```python
from build123d import *

# Parameters (mm, degrees)
BOX011_W          = 9.2
BOX011_H          = 10
BOX011_DEPTH      = 3.4
FILLET005_R       = 1
BOX010_W          = 5.2
BOX010_H          = 50
BOX010_DEPTH      = 1.6
BOX008_W          = 57.2
BOX008_H          = 38.2
BOX008_DEPTH      = 1.6
CYLINDER012_R     = 16.7
CYLINDER012_DEPTH = 1.6
CYLINDER011_R     = 19.9
CYLINDER011_DEPTH = 17
BOX007_W          = 77.1
BOX007_H          = 39.8
BOX007_DEPTH      = 17
CYLINDER010_R     = 21.5
CYLINDER010_DEPTH = 17
BOX006_W          = 78.7
BOX006_H          = 43
BOX006_DEPTH      = 17
FILLET002_R       = 2.4
CHAMFER005_SIZE   = 0.8
CHAMFER013_SIZE   = 0.8


with BuildPart() as usb:
    # Box011 → Box011 (new body)
    with BuildSketch(Plane(origin=(56.4, 45, 9.4), x_dir=(1, 0, 0), z_dir=(0, 0, 1))):
        with Locations((4.6, 5)):
            Rectangle(BOX011_W, BOX011_H)
    extrude(amount=BOX011_DEPTH)

    # Fillet005
    fillet005_edges = [usb.edges().sort_by_distance(p)[0] for p in [
        (56.4, 50, 12.8),
        (56.4, 50, 9.4),
        (65.6, 50, 12.8),
        (65.6, 50, 9.4),
    ]]
    fillet(fillet005_edges, radius=FILLET005_R)


with BuildPart() as obj1:
    # Box010 → Box010 (new body)
    with BuildSketch(Plane(origin=(37.9, 45, 13.8), x_dir=(1, 0, 0), z_dir=(0, 0, 1))):
        with Locations((2.6, 25)):
            Rectangle(BOX010_W, BOX010_H)
    extrude(amount=BOX010_DEPTH)


with BuildPart() as obj2:
    # Box008 → Box008 (new body)
    with BuildSketch(Plane(origin=(0, 50, 0), x_dir=(1, 0, 0), z_dir=(0, 0, 1))):
        with Locations((28.6, 19.1)):
            Rectangle(BOX008_W, BOX008_H)
    extrude(amount=BOX008_DEPTH)


with BuildPart() as zylinder012:
    # Cylinder012 → Cylinder012 (new body)
    with BuildSketch(Plane(origin=(76.2, 69.1, 0), x_dir=(1, 0, 0), z_dir=(0, 0, 1))):
        Circle(CYLINDER012_R)
    extrude(amount=CYLINDER012_DEPTH)


with BuildPart() as zylinder011:
    # Cylinder011 → Cylinder011 (new body)
    with BuildSketch(Plane(origin=(76.2, 69.1, 1.6), x_dir=(1, 0, 0), z_dir=(0, 0, 1))):
        Circle(CYLINDER011_R)
    extrude(amount=CYLINDER011_DEPTH)


with BuildPart() as fusion009:
    # Box007 → Box007 (new body)
    with BuildSketch(Plane(origin=(-0.8, 49.2, 1.6), x_dir=(1, 0, 0), z_dir=(0, 0, 1))):
        with Locations((38.55, 19.9)):
            Rectangle(BOX007_W, BOX007_H)
    extrude(amount=BOX007_DEPTH)

    # Fusion009: union Zylinder011
    add(zylinder011.part)


with BuildPart() as zylinder010:
    # Cylinder010 → Cylinder010 (new body)
    with BuildSketch(Plane(origin=(76.2, 69.1, 0), x_dir=(1, 0, 0), z_dir=(0, 0, 1))):
        Circle(CYLINDER010_R)
    extrude(amount=CYLINDER010_DEPTH)


with BuildPart() as top:
    # Box006 → Box006 (new body)
    with BuildSketch(Plane(origin=(-2.4, 47.6, 0), x_dir=(1, 0, 0), z_dir=(0, 0, 1))):
        with Locations((39.35, 21.5)):
            Rectangle(BOX006_W, BOX006_H)
    extrude(amount=BOX006_DEPTH)

    # Fusion008: union Zylinder010
    add(zylinder010.part)

    # Cut004: cut Fusion009
    add(fusion009.part, mode=Mode.SUBTRACT)

    # Fillet002
    fillet002_edges = [top.edges().sort_by_distance(p)[0] for p in [
        (-2.4, 47.6, 8.5),
        (-2.4, 90.6, 8.5),
    ]]
    fillet(fillet002_edges, radius=FILLET002_R)

    # Cut005: cut Zylinder012
    add(zylinder012.part, mode=Mode.SUBTRACT)

    # Cut006: cut obj2
    add(obj2.part, mode=Mode.SUBTRACT)

    # Chamfer005
    chamfer005_edges = [top.edges().sort_by_distance(p)[0] for p in [
        (57.2, 83.681153, 0),
        (28.6, 88.2, 0),
        (0, 69.1, 0),
        (28.6, 50, 0),
        (57.2, 54.518847, 0),
        (57.2, 69.1, 0),
    ]]
    chamfer(chamfer005_edges, length=CHAMFER005_SIZE)

    # Cut011: cut obj1
    add(obj1.part, mode=Mode.SUBTRACT)

    # Cut018: cut USB
    add(usb.part, mode=Mode.SUBTRACT)

    # Chamfer013
    chamfer013_edges = [top.edges().sort_by_distance(p)[0] for p in [
        (56.692893, 49.2, 12.507107),
        (61, 49.2, 12.8),
        (65.307107, 49.2, 12.507107),
        (65.6, 49.2, 11.1),
        (65.307107, 49.2, 9.692893),
        (61, 49.2, 9.4),
        (56.692893, 49.2, 9.692893),
        (56.4, 49.2, 11.1),
    ]]
    chamfer(chamfer013_edges, length=CHAMFER013_SIZE)


solid = top.part
```
Geometry check sheet. Reference: the model listing, model coordinates, mm. A direction names the side the tool comes from. Coordinates: 2 decimals unless noted, no trailing zeros. Order: outer loops, then holes, each group sorted by start corner. A loop starts at its lowest first (then second) coordinate and runs counter-clockwise, first axis right, second up.
Item 1: Mould release check, pull along X, two halves, no side actions. Record for faces 4 (the flat face through (38, 90.6, 8)), 5 (the cylindrical face through (96.095, 68.664, 9.192)), 6 (the flat face through (-2.4, 69, 8)), 7 (the conical face through (56.459, 48.717, 12.721)): released by +X, released by -X, zero draft, split by the parting line, or undercut.
Item 2: Section check A-A (y = 69.1). Enter the section's corners in (x, z).
Item 3: Section check D-D (x = 75). Enter the section's corners in (y, z).
Item 4: Section check B-B (x = 40). Enter the section's corners in (y, z).
Item 5: Depth check by flat-ended pin: pin 1 (1.3 mm diameter, centred on y = 48.5, z = 14.5, fed in from -X); pin 2 (5 mm diameter, centred on y = 86, z = 8.5, fed in from +X); pin 3 (6 mm diameter, centred on y = 82, z = 4, fed in from +X). Enter the tip coordinate at first touch or a pass-through.
Item 6: Scan lines: line 1 along Y through (x, z) = (23, 9.5); line 2 along X through (y, z) = (69, 6.25); line 3 along Y through (x, z) = (76.2, 0.95). Record each from-to range of solid material in increasing order.
Item 7: Tool access check on faces 1 (the conical face through (65.521, 48.717, 12.741)), 2 (the flat face through (58, 72, 1.6)), 3 (the cylindrical face through (97.695, 68.629, 8.381)). Record the directions out of +Z, -Z, +X, -X, +Y, -Y that give a thin tool (end or side, any length) a straight path to the whole face; none if there is none.
Check sheet entries:
1. face 4: zero draft
1. face 5: undercut
1. face 6: released by -X
1. face 7: undercut
2. outline: (-2.4, 0) - (-0.8, 0) - (0, 0.8) - (0, 1.6) - (-0.8, 1.6) - (-0.8, 17) - (-2.4, 17) - close; (57.2, 0.8) - (58, 0) - (59.5, 0) - (59.5, 1.6) - (57.2, 1.6) - close; (92.9, 0) - (97.7, 0) - (97.7, 17) - (96.1, 17) - (96.1, 1.6) - (92.9, 1.6) - close
3. outline: (47.6, 0) - (52.44, 0) - (52.44, 1.6) - (49.2, 1.6) - (49.2, 17) - (47.6, 17) - close; (85.76, 0) - (90.6, 0) - (90.6, 17) - (89, 17) - (89, 1.6) - (85.76, 1.6) - close
4. outline: (47.6, 0) - (49.2, 0) - (50, 0.8) - (50, 1.6) - (49.2, 1.6) - (49.2, 13.8) - (47.6, 13.8) - close; (47.6, 15.4) - (49.2, 15.4) - (49.2, 17) - (47.6, 17) - close; (88.2, 0.8) - (89, 0) - (90.6, 0) - (90.6, 13.8) - (89, 13.8) - (89, 1.6) - (88.2, 1.6) - close; (89, 15.4) - (90.6, 15.4) - (90.6, 17) - (89, 17) - close
5. pin 1: stops at x = -2.24
5. pin 2: stops at x = 92.17
5. pin 3: stops at x = 95.29
6. line 1: y = 47.6 to 49.2, 89 to 90.6
6. line 2: x = -2.4 to -0.8, 96.1 to 97.7
6. line 3: y = 47.6 to 52.4, 85.8 to 90.6
7. face 1: none
7. face 2: +Z
7. face 3: +Z, -Z, +X
